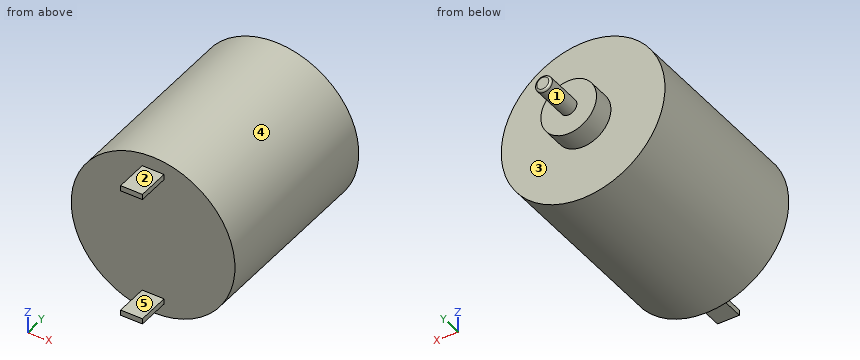
from build123d import *

# Parameters (mm, degrees)
SKETCH_1_R      = 7.5
EXTRUDE_1_DEPTH = 17.2
SKETCH_2_R      = 2.55
EXTRUDE_2_DEPTH = 2
SKETCH_3_R      = 0.75
EXTRUDE_3_DEPTH = 3.6
SKETCH_4_W      = 2
SKETCH_4_H      = 0.5
EXTRUDE_4_DEPTH = 3
FILLET_2_R      = 0.2


with BuildPart() as part:
    # 草圖1 → 伸長1 (new body)
    with BuildSketch(Plane(origin=(0, 0, 0), x_dir=(1, 0, 0), z_dir=(0, 1, 0))):
        with Locations(Location((0, 0, 0), (0, 0, 90))):
            Circle(SKETCH_1_R)
    extrude(amount=EXTRUDE_1_DEPTH)

    # 草圖2 → 伸長2 (add)
    with BuildSketch(Plane(origin=(0, 17.2, 0), x_dir=(1, 0, 0), z_dir=(0, 1, 0))):
        with Locations(Location((0, 0, 0), (0, 0, 270))):
            Circle(SKETCH_2_R)
    extrude(amount=EXTRUDE_2_DEPTH)

    # 草圖3 → 伸長3 (add)
    with BuildSketch(Plane(origin=(0, 19.2, 0), x_dir=(-1, 0, 0), z_dir=(0, 1, 0))):
        with Locations(Location((0, 0, 0), (0, 0, 90))):
            Circle(SKETCH_3_R)
    extrude(amount=EXTRUDE_3_DEPTH)

    # 草圖4 → 伸長4 (add)
    with BuildSketch(Plane.XZ):
        with Locations((0, 6)):
            Rectangle(SKETCH_4_W, SKETCH_4_H)
        with Locations((0, -6)):
            Rectangle(SKETCH_4_W, SKETCH_4_H)
    extrude(amount=EXTRUDE_4_DEPTH)

    # 圓角2
    fillet_2_edges = [part.edges().sort_by_distance(p)[0] for p in [
        (0, 22.8, -0.75),
    ]]
    fillet(fillet_2_edges, radius=FILLET_2_R)


solid = part.part
Can you work these out from the model? Positions are in its coordinate system, mm. Face numbers are marked on the shaded views. A direction names the side the tool comes from. Coordinates: 2 decimals unless noted, no trailing zeros. Loops run counter-clockwise (first coordinate to the right, second up) from the corner with the lowest first, then second, coordinate; pieces in that order, holes last. Notation, with made-up numbers: M 54,47.25 L 108,47.25 A27 cw 108,70.25 Z; hole C 26,33 d8. An arc over 180 degrees is marked long. Return JSON: item names as keys, results as strings. Group by question number.
Item 1: I'm going to push flat-ended pins straight in: pin 1 Ø2 at (x, y) = (-0.5, -2) entering from -Z; pin 2 Ø8 at (x, z) = (-3.5, -4.5) entering from +Y; pin 3 Ø4.5 at (x, z) = (-2.5, -1) entering from -Y. Where does each tip first touch, or does it pass through?
Item 2: Imagine slicing it at B-B (x = 0). Please give me the cut outline in (y, z), and give its area (3 significant figures).
Item 3: If I drill on L1, parallel to Y at x = -6.5, z = -0.5; L2, parallel to X at y = -1.25, z = 6; L3, parallel to Z at x = 0.25, y = 5.5, over which ranges is the centre line in solid material (lowest first)? Write a range as from..to.
Item 4: Imagine slicing it at C-C (y = 14). Please give me the cut outline in (x, z), and give its area (3 significant figures).
Item 5: On a 3-axis mill with a long thin cutter (end or side, diameter ignored), from which of +Z, -Z, +X, -X, +Y, -Y can I reach the whole of each face in a straight line? I mean the marked faces 1 and 2. Say none if no direction works.
Item 6: Thinking about a two-plate mould opening in Z: for the marked faces 3, 4 and 5, which applies, released by +Z, released by -Z, zero draft, split by the parting line, or undercut?
Item 7: Imagine slicing it at A-A (z = 0). Please give me the cut outline in (x, y).
Item 8: Imagine slicing it at D-D (z = -1.5). Please give me the cut outline in (x, y).
Verdict:
{
 "1": {"pin 1": "stops at z = -6.25", "pin 2": "stops at y = 19.2", "pin 3": "stops at y = 0"},
 "2": {"outline": "M -3,-6.25 L 0,-6.25 L 0,-7.5 L 17.2,-7.5 L 17.2,-2.55 L 19.2,-2.55 L 19.2,-0.75 L 22.6,-0.75 A0.2 ccw 22.8,-0.55 L 22.8,0.55 A0.2 ccw 22.6,0.75 L 19.2,0.75 L 19.2,2.55 L 17.2,2.55 L 17.2,7.5 L 0,7.5 L 0,6.25 L -3,6.25 L -3,5.75 L 0,5.75 L 0,-5.75 L -3,-5.75 Z", "area": "277 mm^2"},
 "3": {"L1": "y = 0..17.2", "L2": "x = -1..1", "L3": "z = -7.5..7.5"},
 "4": {"outline": "C 0,0 d15", "area": "177 mm^2"},
 "5": {"face 1": "+Y", "face 2": "+Z, +X, -X, -Y"},
 "6": {"face 3": "zero draft", "face 4": "split by the parting line", "face 5": "undercut"},
 "7": {"outline": "M -7.5,0 L 7.5,0 L 7.5,17.2 L 2.55,17.2 L 2.55,19.2 L 0.75,19.2 L 0.75,22.6 A0.2 ccw 0.55,22.8 L -0.55,22.8 A0.2 ccw -0.75,22.6 L -0.75,19.2 L -2.55,19.2 L -2.55,17.2 L -7.5,17.2 Z"},
 "8": {"outline": "M -7.35,0 L 7.35,0 L 7.35,17.2 L 2.06,17.2 L 2.06,19.2 L -2.06,19.2 L -2.06,17.2 L -7.35,17.2 Z"}
}
